from build123d import *

# Parameters (mm, degrees)
SKETCH3_R               = 25
SKETCH3_R_2             = 22
CUT_EXTRUDE2_DEPTH      = 26
CUT_EXTRUDE2_DEPTH_BACK = 26


with BuildPart() as part:
    # Sweep1: sweep along a path in Sketch1
    with BuildLine(Plane(origin=(0, 0, 0), x_dir=(0, 0, -1), z_dir=(1, 0, 0))) as sweep1_path:
        Line((0, 0), (80, 0))
        Line((80, 0), (92.155372437, 68.936542711))
    # Sketch3 → Sweep1 (sweep)
    with BuildSketch(Plane.XY):
        Circle(SKETCH3_R)
        Circle(SKETCH3_R_2, mode=Mode.SUBTRACT)
    sweep(path=sweep1_path.line, transition=Transition.RIGHT)

    # Sketch4 → Cut-Extrude2 (cut, two sides)
    with BuildSketch(Plane(origin=(0, 0, 0), x_dir=(0, 0, -1), z_dir=(1, 0, 0))) as cut_extrude2_sk:
        Polygon((110.842308967, 30.946164041), (113.687194162, 47.080309724), (94.794337041, 50.411630176), (84.524899127, 52.222409157), (80.652201417, 36.269494553), align=None)
    extrude(amount=CUT_EXTRUDE2_DEPTH, mode=Mode.SUBTRACT)
    extrude(cut_extrude2_sk.sketch, amount=-CUT_EXTRUDE2_DEPTH_BACK, mode=Mode.SUBTRACT)


solid = part.part
Input: part model. Units: mm. Frame: model coordinates. A direction names the side the tool comes from. Coordinates: 2 decimals unless noted, no trailing zeros. Loops run counter-clockwise (first coordinate to the right, second up) from the corner with the lowest first, then second, coordinate; pieces in that order, holes last.
Q1. Set-up query: faces 1 (the face through (1.7, -22.1, 0)), 2 (the face through (11.83, -18.55, -38.98)), 3 (the face through (-1.97, 31.45, -107.98)). Return all of +Z, -Z, +X, -X, +Y, -Y with unobstructed straight access to the full face (end or side cutting, diameter ignored); none if empty.
Q2. Draft query along Z for faces 4 (the face through (22.893, 44.358, -82.616)), 5 (the face through (-22.893, 44.358, -82.616)), 6 (the face through (-22.106, 68.635, -93.864)), 7 (the face through (-3.255, 30.417, -110.533)). Return one class per face: +Z half, -Z half, draft (parallel to the pull), parting line (faces both ways), or undercut.
Q3. Cut plane C-C (x = 2.5). Output: boundary loops of the cut face in (y, z), then the cut area to 3 significant figures.
Q4. Contact query for flat-ended pins moving along their axis: pin 1 (1 mm diameter, centred on x = -16.5, y = 36, fed in from +Z); pin 2 (6 mm diameter, centred on x = 8.5, y = -5, fed in from -Z); pin 3 (12 mm diameter, centred on x = 0.5, y = -6.5, fed in from +Z). Output: stop coordinate, or through.
Q5. Material intervals for line 1 (X direction, y = 0, z = -69); line 2 (X direction, y = 68, z = -97), sorted ascending.
Q6. Cut plane B-B (z = -13). Output: boundary loops of the cut face in (x, y).
Q7. Cut plane A-A (x = -8). Output: boundary loops of the cut face in (y, z).
Working result:
1. face 1: +Z, +X, -X, +Y, -Y
1. face 2: +Z
1. face 3: -Z, +X, -X
2. face 4: undercut
2. face 5: undercut
2. face 6: -Z half
2. face 7: parting line
3. outline: (-24.87, -100.87) - (30.97, -110.72) - (31.49, -107.75) - (-21.86, -98.34) - (-21.86, 0) - (-24.87, 0) - close; (21.86, -61.66) - (72.73, -70.63) - (73.26, -67.66) - (24.87, -59.13) - (24.87, 0) - (21.86, 0) - close; (47.1, -113.56) - (64.62, -116.65) - (65.14, -113.68) - (47.63, -110.59) - close
3. area: 856 mm2
4. pin 1: stops at z = -66.83
4. pin 2: stops at z = -104.05
4. pin 3: stops at z = -99.9
5. line 1: x = -25 to -22, 22 to 25
5. line 2: x = -24.51 to -21.44, 21.44 to 24.51
6. outline: circle Ø50 at (0, 0); hole circle Ø44 at (0, 0)
7. outline: (-23.69, -99.87) - (31.17, -109.55) - (31.73, -106.4) - (-20.49, -97.2) - (-20.49, 0) - (-23.69, 0) - close; (20.49, -62.8) - (72.5, -71.97) - (73.05, -68.83) - (23.69, -60.13) - (23.69, 0) - (20.49, 0) - close; (47.31, -112.39) - (64.82, -115.48) - (65.38, -112.34) - (47.86, -109.25) - close
